Verification items for the finished model (mm, model axes). A direction names the side the tool comes from. Coordinates: 2 decimals unless noted, no trailing zeros. Write each loop counter-clockwise with the first axis right and the second up, starting at its lowest first coordinate (ties: lowest second). Pieces come first, ordered by that corner, then holes. Notation, with made-up numbers: (64.5, -16.5) - (85.5, -16.5) arc R20 cw to (85.5, 1.5) - close; hole circle Ø10 at (64, 51.25). An arc over 180 degrees is marked (long way). Use one line per item in the form item = value. Start each with the question number.
(1) Sectioned sample at A-A (z = 3.5). Record the cut outline in (x, y).
(2) Gauge pin test, flat ends, axial feed: pin 1 Ø1.5 at (x, z) = (1.5, 7) entering from -Y; pin 2 Ø5 at (x, z) = (5.5, 8) entering from +Y; pin 3 Ø2.5 at (x, z) = (7.5, 5) entering from +Y. Record the tip position at first contact, or that the pin passes through.
(3) Sectioned sample at B-B (y = 36). Record the cut outline in (x, z).
(4) Sectioned sample at D-D (z = 1.25). Record the cut outline in (x, y).
(5) Tool access check on faces 1 (the flat face through (6, 26, 9.652)), 2 (the flat face through (6, 35, 7.62)). Record the directions out of +Z, -Z, +X, -X, +Y, -Y that give a thin tool (end or side, any length) a straight path to the whole face; none if there is none.
(6) Material ranges on line 1 (X direction, y = 43, z = 1.75); line 2 (Z direction, x = 4.25, y = 10); line 3 (Z direction, x = 4.25, y = 27), recorded low to high. Write a range as [from, to].
(7) Sectioned sample at C-C (x = 8.5). Record the cut outline in (y, z).
(8) Mould release check, pull along Z, two halves, no side actions. Record for faces 3 (the cylindrical face through (1.06, 29.01, 4.15)), 4 (the flat face through (6, 16, 0)), 5 (the flat face through (6, 23.637, 4)), 6 (the cylindrical face through (5.823, 3.224, 6.928)): released by +Z, released by -Z, zero draft, split by the parting line, or undercut.
from build123d import *

# Parameters (mm, degrees)
SKETCH1_W               = 11.811
SKETCH1_H               = 45.98924
BOSS_EXTRUDE1_DEPTH     = 9.652
FILLET5_R               = 4.826
SKETCH2_W               = 7.62
SKETCH2_H               = 22.352
CUT_EXTRUDE1_DEPTH      = 7.62
CUT_EXTRUDE2_DEPTH      = 49.452771033
CUT_EXTRUDE2_DEPTH_BACK = 49.452771033
SKETCH3_R               = 2.20345
FILLET4_R               = 4.826
FILLET6_R               = 10.16


with BuildPart() as part:
    # Sketch1 → Boss-Extrude1 (new body)
    with BuildSketch(Plane.XY):
        with Locations((5.9055, 22.99462)):
            Rectangle(SKETCH1_W, SKETCH1_H)
    extrude(amount=BOSS_EXTRUDE1_DEPTH)

    # Fillet5
    fillet5_edges = [part.edges().sort_by_distance(p)[0] for p in [
        (5.9055, 45.98924, 0),
    ]]
    fillet(fillet5_edges, radius=FILLET5_R)

    # Sketch2 → Cut-Extrude1 (cut)
    with BuildSketch(Plane(origin=(0, 0, 0), x_dir=(-1, 0, 0), z_dir=(0, 0, -1))):
        with Locations((-5.9055, 34.81324)):
            Rectangle(SKETCH2_W, SKETCH2_H)
    extrude(amount=-CUT_EXTRUDE1_DEPTH, mode=Mode.SUBTRACT)

    # Sketch3 → Cut-Extrude2 (cut, two sides: drawn at the far end of the back side and taken through both)
    with BuildSketch(Plane.ZY.offset(-CUT_EXTRUDE2_DEPTH_BACK)):
        with Locations((4.4323, 26.82494)):
            Circle(SKETCH3_R)
    extrude(amount=CUT_EXTRUDE2_DEPTH + CUT_EXTRUDE2_DEPTH_BACK, mode=Mode.SUBTRACT)

    # Fillet4
    # the kernel refuses this fillet: 4.826 mm, written as the material it takes off along each edge
    with BuildSketch(Plane(origin=(23.876, 45.98924, 9.652), x_dir=(0, 0, -1), z_dir=(-1, 0, 0))) as fillet4_piece_1:
        with BuildLine():
            CenterArc((FILLET4_R, FILLET4_R), FILLET4_R, 180, 90)
            Line((0, FILLET4_R), (0, 0))
            Line((0, 0), (FILLET4_R, 0))
        make_face()
    extrude(amount=35.941, mode=Mode.SUBTRACT)

    # Fillet6
    # the kernel refuses this fillet: 10.16 mm, written as the material it takes off along each edge
    with BuildSketch(Plane(origin=(-25.368230131, 0, 9.652), x_dir=(0, 1, 0), z_dir=(1, 0, 0))) as fillet6_piece_1:
        with BuildLine():
            CenterArc((10.147292053, -10.16), FILLET6_R, 90, 87.134016017)
            Line((0, -9.652), (-0.202945841, -9.64184))
            ThreePointArc((-0.202945841, -9.64184), (-0.2032, -4.826), (-0.2032, 0))
            Line((-0.2032, 0), (0, 0.2032))
            Line((0, 0.2032), (10.147292053, 0.2032))
            Line((10.147292053, 0.2032), (10.147292053, 0))
        make_face()
    extrude(amount=62.547460263, mode=Mode.SUBTRACT)


solid = part.part
Answers below:
q1.outline = (0, 0.81) - (11.81, 0.81) - (11.81, 24.83) - (9.72, 24.83) - (9.72, 23.64) - (2.1, 23.64) - (2.1, 24.83) - (0, 24.83) - close; (0, 28.82) - (2.1, 28.82) - (2.1, 45.8) - (0, 45.8) - close; (9.72, 28.82) - (11.81, 28.82) - (11.81, 45.8) - (9.72, 45.8) - close
q2.pin_1 = 2.56
q2.pin_2 = 45.1
q2.pin_3 = 23.64
q3.outline = (0, 0) - (2.1, 0) - (2.1, 7.62) - (9.72, 7.62) - (9.72, 0) - (11.81, 0) - (11.81, 9.65) - (0, 9.65) - close
q4.outline = (0, 0.14) - (11.81, 0.14) - (11.81, 44.4) - (9.72, 44.4) - (9.72, 23.64) - (2.1, 23.64) - (2.1, 44.4) - (0, 44.4) - close
q5.face_1 = +Z, +X, -X, +Y, -Y
q5.face_2 = -Z, +Y
q6.line_1 = [0, 2.1], [9.72, 11.81]
q6.line_2 = [0, 9.65]
q6.line_3 = [7.62, 9.65]
q7.outline = (0, 0) - (23.64, 0) - (23.64, 7.62) - (45.1, 7.62) arc R4.83 ccw to (41.16, 9.65) - (10.15, 9.65) arc R10.16 ccw to start
q8.face_3 = undercut
q8.face_4 = released by -Z
q8.face_5 = zero draft
q8.face_6 = released by +Z
